Verification items for the finished model (mm, model axes). Face numbers are marked on the shaded views. A direction names the side the tool comes from. Coordinates: 2 decimals unless noted, no trailing zeros. Order: outer loops, then holes, each group sorted by start corner. A loop starts at its lowest first (then second) coordinate and runs counter-clockwise, first axis right, second up. Notation, with made-up numbers: M -40,65.25 L -14,65.25 A38 ccw -14,104.25 Z; hole C 18.5,26 d11. An arc over 180 degrees is marked long. Answer as a JSON object with one key per item and string values. Group by question number.
(1) Material ranges on line 1 (X direction, y = 66, z = 8.75); line 2 (Z direction, x = 74, y = 24.5); line 3 (Z direction, x = 29.5, y = 6), recorded low to high.
(2) Mould release check, pull along X, two halves, no side actions. Record for the marked faces 1, 2, 3 and 4: released by +X, released by -X, zero draft, split by the parting line, or undercut.
(3) Gauge pin test, flat end, axial feed: pin 1 Ø9 at (x, y) = (47.5, 57) entering from +Z. Record the tip position at first contact, or that the pin passes through.
(4) Cross-section at A-A (z = 12.5). Enter the section's corners in (x, y), plus the area to 3 significant figures.
(5) Cross-section at C-C (x = 37.5). Enter the section's corners in (y, z), plus the area to 3 significant figures.
(6) Cross-section at B-B (y = 22.5). Enter the section's corners in (x, z), plus the area to 3 significant figures.
(7) Access from +Z, -Z, +X, -X, +Y, -Y to the whole of each face (thin tool, end or side, straight path). Record for the marked faces 5 and 6.
(8) Cross-section at D-D (x = 75). Enter the section's corners in (y, z), plus the area to 3 significant figures.
from build123d import *

# Parameters (mm, degrees)
F0_W     = 101.6
F0_H     = 76.2
F1_DEPTH = 15.24
F2_W     = 3.048
F2_H     = 76.2
F3_DEPTH = 9.144
F4_W     = 30.48
F4_H     = 76.2
F5_DEPTH = 10.16
F6_W     = 7.366
F6_H     = 76.2
F7_DEPTH = 17.78


with BuildPart() as f1:
    # F0 (on Top) → F1 (new body)
    with BuildSketch(Plane.XY):
        with Locations((50.8, 38.1)):
            Rectangle(F0_W, F0_H)
    extrude(amount=F1_DEPTH)

    # F2 (on face) → F3 (cut)
    with BuildSketch(Plane.XY.offset(15.24)):
        with Locations((74.676, 38.1)):
            Rectangle(F2_W, F2_H)
    extrude(amount=-F3_DEPTH, mode=Mode.SUBTRACT)

    # F4 (on face) → F5 (cut)
    with BuildSketch(Plane.XY.offset(15.24)):
        with Locations((42.672, 38.1)):
            Rectangle(F4_W, F4_H)
    extrude(amount=-F5_DEPTH, mode=Mode.SUBTRACT)

    # F6 (on face) → F7 (cut)
    with BuildSketch(Plane.XY.offset(15.24)):
        with Locations((3.683, 38.1)):
            Rectangle(F6_W, F6_H)
    extrude(amount=-F7_DEPTH, mode=Mode.SUBTRACT)


solid = f1.part
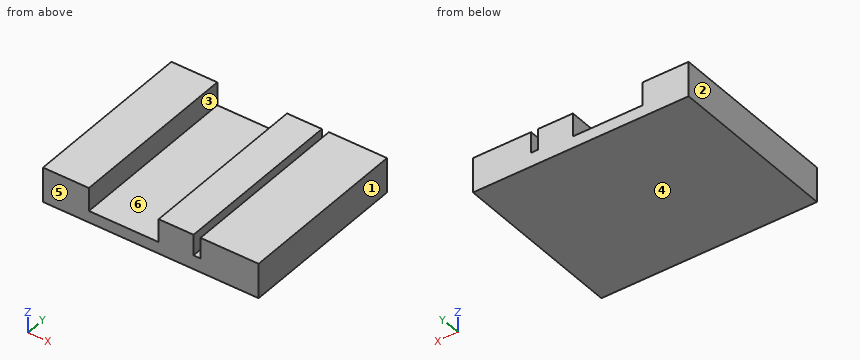
Taken from the geometry:
{
 "1": {"line 1": "x = 7.37 to 27.43, 57.91 to 73.15, 76.2 to 101.6", "line 2": "z = 0 to 6.1", "line 3": "z = 0 to 5.08"},
 "2": {"face 1": "released by +X", "face 2": "released by -X", "face 3": "undercut", "face 4": "zero draft"},
 "3": {"pin 1": "stops at z = 5.08"},
 "4": {"outline": "M 7.37,0 L 27.43,0 L 27.43,76.2 L 7.37,76.2 Z; M 57.91,0 L 73.15,0 L 73.15,76.2 L 57.91,76.2 Z; M 76.2,0 L 101.6,0 L 101.6,76.2 L 76.2,76.2 Z", "area": "4,630 mm²"},
 "5": {"outline": "M 0,0 L 76.2,0 L 76.2,5.08 L 0,5.08 Z", "area": "387 mm²"},
 "6": {"outline": "M 7.37,0 L 101.6,0 L 101.6,15.24 L 76.2,15.24 L 76.2,6.1 L 73.15,6.1 L 73.15,15.24 L 57.91,15.24 L 57.91,5.08 L 27.43,5.08 L 27.43,15.24 L 7.37,15.24 Z", "area": "1,100 mm²"},
 "7": {"face 5": "+Z, -Z, +X, -X, -Y", "face 6": "+Z, +Y, -Y"},
 "8": {"outline": "M 0,0 L 76.2,0 L 76.2,6.1 L 0,6.1 Z", "area": "465 mm²"}
}
